Geometry: final body of the model. Coordinates: model frame, mm. A direction names the side the tool comes from. Give positions to 0.01 mm unless a question says otherwise; leave off trailing zeros. Loops run counter-clockwise (first coordinate to the right, second up) from the corner with the lowest first, then second, coordinate; pieces in that order, holes last.
1. Material intervals for line 1 along Y through (x, z) = (0, 2) (3 decimals); line 2 along Y through (x, z) = (0, 95); line 3 along X through (y, z) = (5.25, 57.5), sorted ascending.
2. Draft query along Y for faces 1 (the face through (-13, -1, 3.175)), 2 (the face through (3.6, 1.13, 6.95)), 3 (the face through (-2.75, 12.4, 1.69)), 4 (the face through (-0.69, 3.1, 3.13)). Return one class per face: +Y half, -Y half, draft (parallel to the pull), parting line (faces both ways), or undercut.
3. First-contact query: P1, Ø1.5, axis at y = 7, z = 44.5, coming from the +X side; P2, Ø6, axis at y = 7, z = 97, coming from the -X side; P3, Ø1.5, axis at y = 8.5, z = 161, coming from the +X side. Flat tips, straight axial feed; report the tip coordinate or a pass-through.
4. Section C-C, the plane z = 37.5. Output: boundary loops of the cut face in (x, y) (1 decimal).
5. Access query for faces 5 (the face through (-2.75, 12.4, 97.27)), 6 (the face through (-13, -1, 180.975)). Directions: +Z, -Z, +X, -X, +Y, -Y. A direction counts if a zero-diameter tool reaches every point of the face in a straight line with its end or side. Return the directions, or none.
Autodesk Inventor part; units mm, degrees
ref_plane "YZ Plane" through (0, 0, 0) normal (1, 0, 0) x (0, 1, 0)
ref_plane "XZ Plane" through (0, 0, 0) normal (0, 1, 0) x (-1, 0, 0)
ref_plane "XY Plane" through (0, 0, 0) normal (0, 0, 1) x (1, 0, 0)
sketch "Sketch1" plane through (0, 0, 0) normal (0, 0, 1) x (1, 0, 0)
  circle A0 centre (0, 0) radius 12.7
  circle A1 centre (0, 0) radius 3.175
  dimension "d0" = 6.35
extrude "Extrusion1" add sketch "Sketch1" along normal blind 3.175
sketch "Sketch2" plane through (0, 0, 3.175) normal (0, 0, 1) x (1, 0, 0)
  circle A0 centre (0, 0) radius 12.7
  circle A1 centre (0, 0) radius 11.1125
  circle A2 centre (0, 0) radius 14.2875
  dimension "d3" = 22.225
  dimension "d4" = 28.575
extrude "Extrusion2" add sketch "Sketch2" along normal blind 177.8 contours A2
sketch "Sketch3" plane through (0, 0, 3.175) normal (0, 0, 1) x (1, 0, 0)
  circle A0 centre (0, 0) radius 12.7
  circle A1 centre (0, 0) radius 3.175
extrude "Extrusion3" add sketch "Sketch3" along normal blind 3.175
chamfer "Chamfer1" distance 9.525 angle 45 1 edges at (-12.7, 0, 6.35)
chamfer "Chamfer2" distance 0.254 angle 45 1 edges at (-12.7, 0, 0)
properties part number "pourTool"
Answers below:
1. line 1: y = -12.7 to -3.175, 3.175 to 12.7
1. line 2: y = -14.29 to -12.7, 12.7 to 14.29
1. line 3: x = -13.29 to -11.56, 11.56 to 13.29
2. face 1: draft
2. face 2: undercut
2. face 3: parting line
2. face 4: undercut
3. P1: stops at x = 12.85
3. P2: stops at x = -13.72
3. P3: stops at x = 12
4. outline: circle Ø28.6 at (0, 0); hole circle Ø25.4 at (0, 0)
5. face 5: +Z
5. face 6: +Z, +X, -X, +Y, -Y
